Here's how the part is built. I have some questions about the finished solid (model axes, mm). Face numbers are marked on the shaded views. A direction names the side the tool comes from. Give positions to 0.01 mm unless a question says otherwise; leave off trailing zeros. Loops run counter-clockwise (first coordinate to the right, second up) from the corner with the lowest first, then second, coordinate; pieces in that order, holes last.
Q1. If we section it at A-A (y = 2.5): Please give me the cut outline in (x, z), plus the area to 4 significant figures.
Q2. If we section it at B-B (x = -13.5): Please give me the cut outline in (y, z).
Q3. I need wall thicknesses on line 1 (Y direction, x = -9, z = 18); line 2 (Z direction, x = -4, y = 18); line 3 (X direction, y = 18.25, z = 13.25). Which ranges of each line are inside material? Lowest first, please.
Q4. For the marked faces 1, 2 and 3, which set-ups out of +Z, -Z, +X, -X, +Y, -Y let a thin tool reach every point of the face, with its end or its side?
Q5. If we section it at D-D (y = 7.5): Please give me the cut outline in (x, z), plus the area to 4 significant figures.
Q6. Will these pins go through, and if not, where does the flat tip stop? P1, Ø1.5, axis at x = -16.5, y = 1.5, coming from the +Z side; P2, Ø2.5, axis at y = 17.5, z = 13, coming from the -X side; P3, Ø5, axis at y = 11, z = 17, coming from the -X side.
Q7. If we section it at C-C (z = 13): Please give me the cut outline in (x, y).
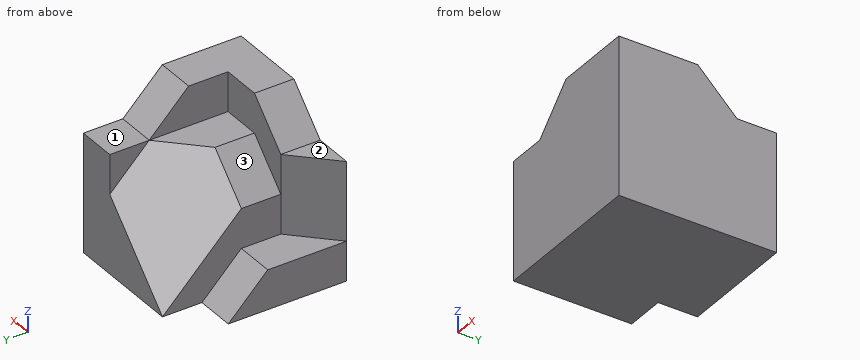
from build123d import *

# Parameters (mm, degrees)
BOSS_EXTRUDE1_DEPTH = 20
SKETCH2_W           = 5
SKETCH2_H           = 15
BOSS_EXTRUDE3_DEPTH = 5
CUT_EXTRUDE2_DEPTH  = 5
BOSS_EXTRUDE4_DEPTH = 20
CUT_EXTRUDE3_DEPTH  = 37
BOSS_EXTRUDE5_DEPTH = 5
SKETCH7_W           = 5
SKETCH7_H           = 5
BOSS_EXTRUDE6_DEPTH = 10
CUT_EXTRUDE4_DEPTH  = 10
BOSS_EXTRUDE7_DEPTH = 5


with BuildPart() as part:
    # Sketch1 → Boss-Extrude1 (new body)
    with BuildSketch(Plane(origin=(0, 0, 0), x_dir=(1, 0, 0), z_dir=(0, 1, 0))):
        Polygon((-15, 0), (0, 0), (0, -15), (-5, -15), (-5, -10), align=None)
    extrude(amount=BOSS_EXTRUDE1_DEPTH)

    # Sketch2 → Boss-Extrude3 (add)
    with BuildSketch(Plane.XY.offset(15)):
        with Locations((-2.5, 7.5)):
            Rectangle(SKETCH2_W, SKETCH2_H)
    extrude(amount=BOSS_EXTRUDE3_DEPTH)

    # Sketch4 → Cut-Extrude2 (cut)
    with BuildSketch(Plane.ZY.offset(5)):
        Polygon((15, 15), (20, 10), (20, 15), align=None)
    extrude(amount=-CUT_EXTRUDE2_DEPTH, mode=Mode.SUBTRACT)

    # Sketch5 → Boss-Extrude4 (add)
    with BuildSketch(Plane(origin=(0, 0, 0), x_dir=(-1, 0, 0), z_dir=(0, -1, 0))):
        Polygon((15, 0), (15, -10), (10, -15), (5, -15), (5, -10), align=None)
    extrude(amount=-BOSS_EXTRUDE4_DEPTH)

    # 3DSketch1 → Cut-Extrude3 (cut, along a direction that is not the sketch's normal)
    with BuildSketch(Plane(origin=(-15, 20, 0), x_dir=(0.5345224838248489, -0.26726124191242445, 0.8017837257372732), z_dir=(0.5773502691896253, -0.5773502691896264, -0.5773502691896257))):
        Polygon((0, 0), (13.363062096, -4.629100499), (18.708286934, 0), (17.371980724, 6.943650748), (10.690449676, 9.258200998), align=None)
    extrude(amount=-CUT_EXTRUDE3_DEPTH, dir=(0, 0, -1), mode=Mode.SUBTRACT)

    # Sketch6 → Boss-Extrude5 (add)
    with BuildSketch(Plane.ZY.offset(15)):
        Polygon((0, 0), (0, 15), (5, 10), (5, 0), align=None)
    extrude(amount=BOSS_EXTRUDE5_DEPTH)

    # Sketch7 → Boss-Extrude6 (add)
    with BuildSketch(Plane.XY.offset(5)):
        with Locations((-17.5, 2.5)):
            Rectangle(SKETCH7_W, SKETCH7_H)
    extrude(amount=BOSS_EXTRUDE6_DEPTH)

    # Sketch8 → Cut-Extrude4 (cut)
    with BuildSketch(Plane.XY.offset(15)):
        Polygon((-20, 0), (-15, 5), (-20, 5), align=None)
    extrude(amount=-CUT_EXTRUDE4_DEPTH, mode=Mode.SUBTRACT)

    # Sketch9 → Boss-Extrude7 (add)
    with BuildSketch(Plane(origin=(0, 0, 0), x_dir=(-1, 0, 0), z_dir=(0, -1, 0))):
        Polygon((15, -15), (15, -10), (10, -15), (5, -15), (5, -20), (10, -20), align=None)
    extrude(amount=-BOSS_EXTRUDE7_DEPTH)


solid = part.part
Check sheet entries:
1. outline: (-20, 0) - (0, 0) - (0, 20) - (-10, 20) - (-15, 15) - (-17.5, 15) - (-17.5, 5) - (-20, 5) - close
1. area: 337.5 mm2
2. outline: (0, 0) - (20, 0) - (20, 1.5) - (10, 11.5) - (5, 11.5) - (5, 16.5) - (0, 16.5) - close
3. line 1: y = 0 to 5
3. line 2: z = 0 to 15
3. line 3: x = -5 to 0
4. face 1: +Z, +X, -X, +Y
4. face 2: +Z, -X, +Y, -Y
4. face 3: +Z, -X, +Y
5. outline: (-20, 0) - (0, 0) - (0, 20) - (-5, 20) - (-5, 15) - (-10, 15) - (-15, 10) - (-15, 5) - (-20, 5) - close
5. area: 262.5 mm2
6. P1: stops at z = 15
6. P2: stops at x = -6.27
6. P3: stops at x = -10.29
7. outline: (-20, 0) - (0, 0) - (0, 20) - (-5, 20) - (-5, 17) - (-12, 10) - (-12, 5) - (-15, 5) - close
